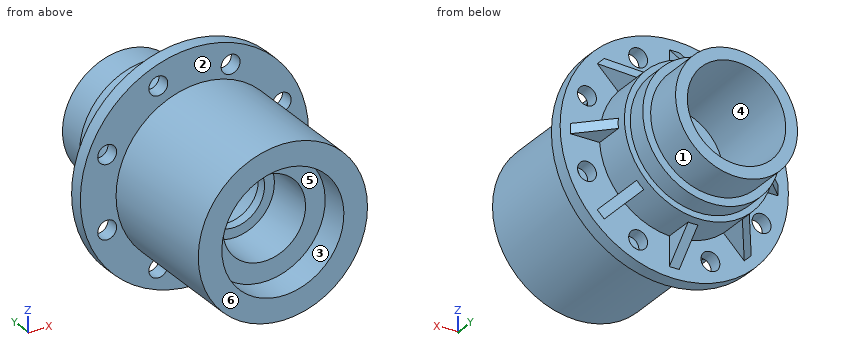
```python
from build123d import *

# Parameters (mm, degrees)
RIB1_REACH         = 292
SKETCH2_WALL_W     = 687.361283212
SKETCH2_WALL_H     = 25
SKETCH3_R          = 24
CUT_EXTRUDE1_DEPTH = 35
CIRPATTERN1_COUNT  = 8
CIRPATTERN2_COUNT  = 8


with BuildPart() as part:
    # Sketch1 → Revolve1 (revolve)
    with BuildSketch(Plane.XY, mode=Mode.PRIVATE) as revolve1_sk:
        Polygon((125, 640), (125, 390), (80, 390), (80, 355), (125, 355), (105, 225), (80, 225), (80, 200), (105, 200), (105, 75), (155, 75), (155, 0), (215, 0), (215, 330), (190, 330), (190, 355), (290, 355), (290, 390), (190, 390), (190, 490), (175, 490), (175, 540), (155, 540), (155, 640), align=None)
    revolve(revolve1_sk.sketch.rotate(Axis((0, 580.752844837, 0), (0, -1, 0)), 90), axis=Axis((0, 580.752844837, 0), (0, -1, 0)))  # turned: the seam where the file's is

    # Sketch2 wall → Rib1 (add, up to next)
    with BuildSketch(Plane(origin=(227, 427.5, 0), x_dir=(-0.70234528, 0.711836433, 0), z_dir=(-0.711836433, -0.70234528, 0)), mode=Mode.PRIVATE) as rib1_sk1:
        Rectangle(SKETCH2_WALL_W, SKETCH2_WALL_H)
    rib1_tool1 = extrude(rib1_sk1.sketch, amount=RIB1_REACH, mode=Mode.PRIVATE) - part.part
    rib1 = rib1_tool1.solids().sort_by_distance((227, 427.5, 0))[0]
    add(rib1)

    # Sketch3 → Cut-Extrude1 (cut)
    with BuildSketch(Plane(origin=(0, 390, 0), x_dir=(1, 0, 0), z_dir=(0, 1, 0))):
        with Locations(Location((221.731087803, 91.844023768, 0), (0, 0, 270))):  # turned: the seam where the file's is
            Circle(SKETCH3_R)
    cut_extrude1 = extrude(amount=-CUT_EXTRUDE1_DEPTH, mode=Mode.SUBTRACT)

    # CirPattern1: Rib1 ×8 about axis
    cirpattern1_axis = Axis((0, 0, 0), (0, 1, 0))
    for i in range(1, CIRPATTERN1_COUNT):
        add(rib1.rotate(cirpattern1_axis, i * 360 / CIRPATTERN1_COUNT))

    # CirPattern2: Cut-Extrude1 ×8 about axis
    cirpattern2_axis = Axis((0, 0, 0), (0, 1, 0))
    for i in range(1, CIRPATTERN2_COUNT):
        add(cut_extrude1.rotate(cirpattern2_axis, i * 360 / CIRPATTERN2_COUNT), mode=Mode.SUBTRACT)


solid = part.part
```
Part model, mm, in its own coordinate system. Face numbers are marked on the shaded views. A direction names the side the tool comes from. Coordinates: 2 decimals unless noted, no trailing zeros. Loops run counter-clockwise (first coordinate to the right, second up) from the corner with the lowest first, then second, coordinate; pieces in that order, holes last. Notation, with made-up numbers: (-3.5, 8.25) - (30.5, 8.25) arc R28 cw to (30.5, 29.25) - close; hole circle Ø2 at (30, 57.25). An arc over 180 degrees is marked (long way). Write item = value, one per line. Start each with the question number.
Item 1: Flat gauge pins, fed straight in: pin 1 Ø2 at (y, z) = (129.5, 69) entering from -X; pin 2 Ø3 at (x, y) = (76, 137) entering from +Z; pin 3 Ø1.5 at (x, y) = (52, 299.5) entering from -Z. Where does each tip first touch, or does it go through?
Item 2: Wall check: L1, parallel to Y at x = -187, z = 55; L2, parallel to Z at x = 0.5, y = 123; L3, parallel to Y at x = -124.5, z = -32. Give the ranges that are in metal, low to high. Write a range as from..to.
Item 3: Cut at A-A, the plane y = 121.5. Give the cut face in (x, z).
Item 4: Cut at B-B, the plane y = 244. Give the cut face in (x, z).
Item 5: Mould opens along Z. For the marked faces 1, 2 and 3 say: released by +Z, released by -Z, zero draft, split by the parting line, or undercut.
Item 6: 3-axis set-ups, long thin cutter, end or side, ignore diameter. For the marked faces 4, 5 and 6: which of +Z, -Z, +X, -X, +Y, -Y reach the whole face in a straight line?
The answers:
q1.pin_1 = -203.96
q1.pin_2 = 201.68
q1.pin_3 = -208.8
q2.L1 = 0..330, 355..390
q2.L2 = -215..-105, 105..215
q2.L3 = 75..640
q3.outline = circle Ø430 at (0, 0); hole circle Ø210 at (0, 0)
q4.outline = circle Ø430 at (0, 0); hole circle Ø215.85 at (0, 0)
q5.face_1 = split by the parting line
q5.face_2 = zero draft
q5.face_3 = undercut
q6.face_4 = +Y
q6.face_5 = -Y
q6.face_6 = +Z, -Z, +X, -X, -Y
